Work out the finished part from the listing and answer in its coordinate system (mm). Face numbers are marked on the shaded views. A direction names the side the tool comes from. Round coordinates to 2 decimals unless told otherwise and drop trailing zeros. Write each loop counter-clockwise with the first axis right and the second up, starting at its lowest first coordinate (ties: lowest second). Pieces come first, ordered by that corner, then holes. Notation, with made-up numbers: (5, 7) -> (56, 7) arc R19 cw to (56, 26) -> close; hole circle Ø4 at (-33.5, 19.5). An arc over 180 degrees is marked (long way). One line per item, written item: value.
```python
from build123d import *

# Parameters (mm, degrees)
ESBO_O1_R                     = 15
RESSALTO_EXTRUS_O1_DEPTH      = 165
ESBO_O3_R                     = 15
RESSALTO_EXTRUS_O2_DEPTH      = 30
RESSALTO_EXTRUS_O2_DEPTH_BACK = 30


with BuildPart() as part:
    # Esbo_o1 → Ressalto-extrus_o1 (new body)
    with BuildSketch(Plane(origin=(0, 0, 0), x_dir=(1, 0, 0), z_dir=(0, 1, 0))):
        Circle(ESBO_O1_R)
    extrude(amount=-RESSALTO_EXTRUS_O1_DEPTH)

    # Esbo_o3 → Ressalto-extrus_o2 (add, two sides)
    with BuildSketch(Plane(origin=(0, 0, 0), x_dir=(0, 0, -1), z_dir=(1, 0, 0))) as ressalto_extrus_o2_sk:
        with Locations((0, -15)):
            Circle(ESBO_O3_R)
    extrude(amount=RESSALTO_EXTRUS_O2_DEPTH)
    extrude(ressalto_extrus_o2_sk.sketch, amount=-RESSALTO_EXTRUS_O2_DEPTH_BACK)


solid = part.part
```
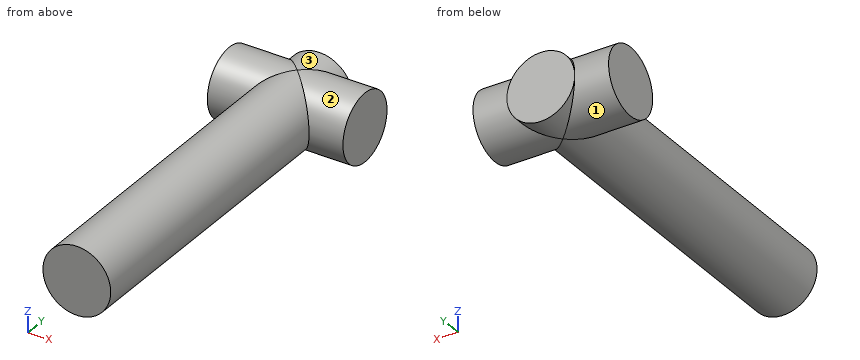
(1) Find section A-A on x = 9. Give the vertices of the cut face in (y, z), plus the area to 3 significant figures.
Reported:
outline: (-165, -12) -> (-24, -12) arc R15 ccw to (-6, -12) -> (0, -12) -> (0, 12) -> (-6, 12) arc R15 ccw to (-24, 12) -> (-165, 12) -> close
area: 4,030 mm2
(2) Find section C-C on y = -64. Give the vertices of the cut face in (x, z), plus the area to 3 significant figures.
Reported:
outline: circle Ø30 at (0, 0)
area: 707 mm2
(3) Find section D-D on x = 19. Give the vertices of the cut face in (y, z).
Reported:
outline: circle Ø30 at (-15, 0)
(4) Consider probe 1 along X at (y, z) = (-111, 0.75); probe 2 along Z at (x, y) = (0, -156.5); probe 3 along X at (y, z) = (-99.5, 7.25). Determine where each line is inside the solid, lowest interval first.
Reported:
probe 1: x = -14.98 to 14.98
probe 2: z = -15 to 15
probe 3: x = -13.13 to 13.13
(5) Flat-ended cylindrical pins translate along their axes: pin 1 Ø10 at (x, z) = (21.5, 10) entering from +Y; pin 2 Ø3 at (x, y) = (12.5, -103.5) entering from -Z; pin 3 Ø2 at (x, y) = (10.5, -115.5) entering from -Z. Find the tip coordinate at first contact, or state that the pin passes through.
Reported:
pin 1: stops at y = -0.86
pin 2: stops at z = -10.2
pin 3: stops at z = -11.61
(6) Find section B-B on z = -8. Give the vertices of the cut face in (x, y), plus the area to 3 significant figures.
Reported:
outline: (-30, -27.69) -> (-12.69, -27.69) -> (-12.69, -165) -> (12.69, -165) -> (12.69, -27.69) -> (30, -27.69) -> (30, -2.31) -> (12.69, -2.31) -> (12.69, 0) -> (-12.69, 0) -> (-12.69, -2.31) -> (-30, -2.31) -> close
area: 5,070 mm2
(7) A tool of negligible diameter and unlimited length cuts with its end or side. For the marked faces 1, 2 and 3, from which of +Z, -Z, +X, -X, +Y, -Y can it reach the whole face along a straight path? Write none if from no direction.
Reported:
face 1: -X
face 2: +X
face 3: +Z, +Y
